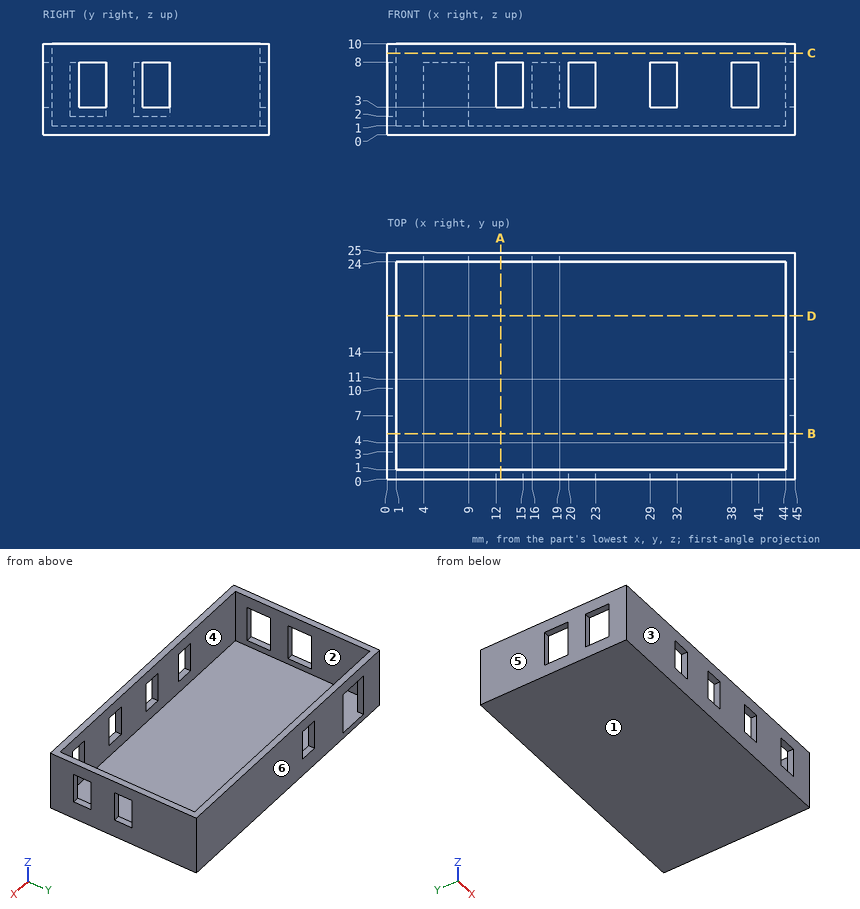
Check sheet for the drawn part. Datum: minimum x, y, z corner. Units: mm. A direction names the side the tool comes from. Coordinates: 2 decimals unless noted, no trailing zeros. Order: outer loops, then holes, each group sorted by start corner. A loop starts at its lowest first (then second) coordinate and runs counter-clockwise, first axis right, second up. Notation, with made-up numbers: (61.5, 45.5) -> (84.5, 45.5) arc R12 cw to (84.5, 54.5) -> close; hole circle Ø4 at (-23.5, 48). An arc over 180 degrees is marked (long way). Write each question's results on one line, items separated by ' | '. Start each with the question number.
1) Section check D-D (y = 18). Enter the section's corners in (x, z), and give its area (3 significant figures).
2) Material ranges on line 1 along X through (y, z) = (2, 8.5); line 2 along Y through (x, z) = (41, 8.5); line 3 along Z through (x, y) = (36.5, 7.75), recorded low to high.
3) Set-up check for the marked faces 1 and 2: record each of +Z, -Z, +X, -X, +Y, -Y from which the full face is reachable in a straight line by a thin tool's end or side.
4) Section check A-A (x = 12.5). Enter the section's corners in (y, z).
5) Section check B-B (y = 5). Enter the section's corners in (x, z).
6) Section check C-C (z = 9). Enter the section's corners in (x, y), and give its area (3 significant figures).
7) Draft check along Y on the marked faces 3, 4, 5 and 6. Enter one of: pulls with the +Y half, pulls with the -Y half, needs draft (parallel to the pull), parting line crosses it, or undercut.
Checked values:
1) outline: (0, 0) -> (45, 0) -> (45, 10) -> (44, 10) -> (44, 1) -> (1, 1) -> (1, 10) -> (0, 10) -> close | area: 63.0 mm²
2) line 1: 0 to 1, 44 to 45 | line 2: 0 to 1, 24 to 25 | line 3: 0 to 1
3) face 1: -Z, +X, -X, +Y, -Y | face 2: +Z
4) outline: (0, 0) -> (25, 0) -> (25, 10) -> (24, 10) -> (24, 1) -> (1, 1) -> (1, 3) -> (0, 3) -> close; (0, 8) -> (1, 8) -> (1, 10) -> (0, 10) -> close
5) outline: (0, 0) -> (45, 0) -> (45, 3) -> (44, 3) -> (44, 1) -> (1, 1) -> (1, 2) -> (0, 2) -> close; (0, 8) -> (1, 8) -> (1, 10) -> (0, 10) -> close; (44, 8) -> (45, 8) -> (45, 10) -> (44, 10) -> close
6) outline: (0, 0) -> (45, 0) -> (45, 25) -> (0, 25) -> close; hole (1, 1) -> (44, 1) -> (44, 24) -> (1, 24) -> close | area: 136 mm²
7) face 3: pulls with the -Y half | face 4: undercut | face 5: needs draft | face 6: pulls with the +Y half
